Here's the drawing with two shaded views (mm, measured from the low corner). I have some questions. Coordinates: 2 decimals unless noted, no trailing zeros. Write each loop counter-clockwise with the first axis right and the second up, starting at its lowest first coordinate (ties: lowest second). Pieces come first, ordered by that corner, then holes.
Item 1: I want a section at C-C on y = 6.5. Please give me the cut outline in (x, z).
Item 2: I want a section at D-D on x = 7.75. Please give me the cut outline in (y, z), then the cut area to 3 significant figures.
Item 3: I want a section at A-A on z = 2.2. Please give me the cut outline in (x, y), then the cut area to 3 significant figures.
Item 4: For P1, Ø1.2, axis at x = 9, z = 2.5, coming from the -Y side; P2, Ø0.6, axis at y = 11.5, z = 2.5, coming from the -X side; P3, Ø0.6, axis at x = 4.5, z = 2, coming from the -Y side, each with a flat end and sliding along its axis, tell me the tip position at first contact or that it passes through.
Item 5: If I drill on probe 1 along Y at (x, z) = (3.5, 1.75); probe 2 along Z at (x, y) = (5.5, 4.5); probe 3 along X at (y, z) = (3.75, 2), over which ranges is the centre line in solid material (lowest first)?
Item 6: I want a section at B-B on x = 16. Please give me the cut outline in (y, z), then the cut area to 3 significant figures.
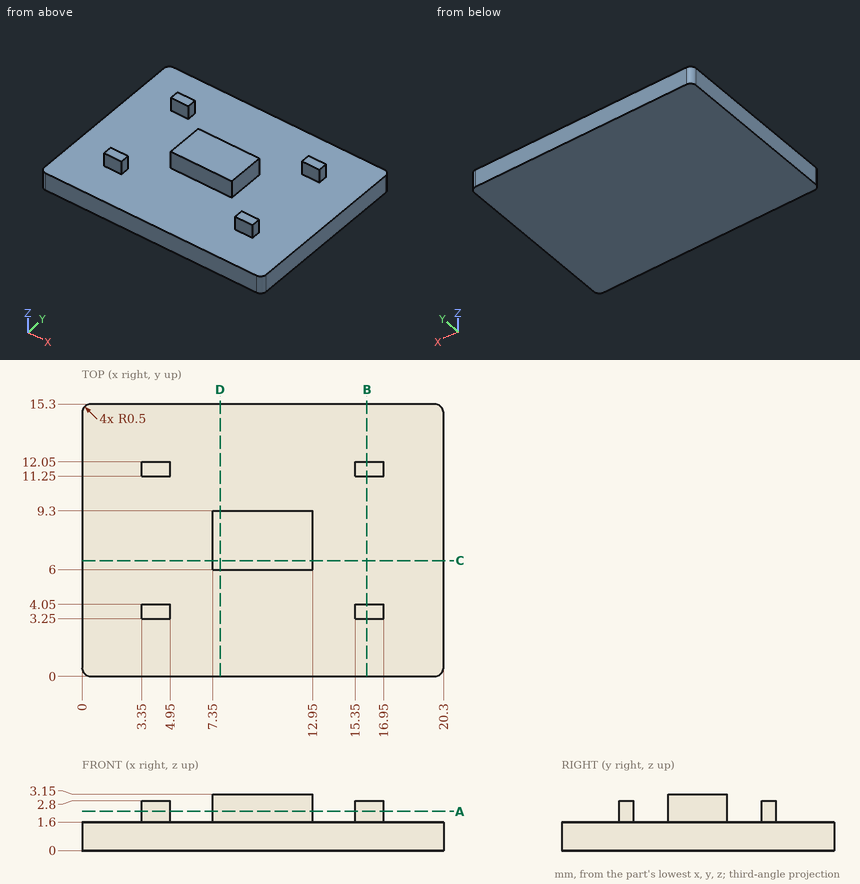
Response values:
1. outline: (0, 0) - (20.3, 0) - (20.3, 1.6) - (12.95, 1.6) - (12.95, 3.15) - (7.35, 3.15) - (7.35, 1.6) - (0, 1.6) - close
2. outline: (0, 0) - (15.3, 0) - (15.3, 1.6) - (9.3, 1.6) - (9.3, 3.15) - (6, 3.15) - (6, 1.6) - (0, 1.6) - close
2. area: 29.6 mm2
3. outline: (3.35, 3.25) - (4.95, 3.25) - (4.95, 4.05) - (3.35, 4.05) - close; (3.35, 11.25) - (4.95, 11.25) - (4.95, 12.05) - (3.35, 12.05) - close; (7.35, 6) - (12.95, 6) - (12.95, 9.3) - (7.35, 9.3) - close; (15.35, 3.25) - (16.95, 3.25) - (16.95, 4.05) - (15.35, 4.05) - close; (15.35, 11.25) - (16.95, 11.25) - (16.95, 12.05) - (15.35, 12.05) - close
3. area: 23.6 mm2
4. P1: stops at y = 6
4. P2: stops at x = 3.35
4. P3: stops at y = 3.25
5. probe 1: y = 3.25 to 4.05, 11.25 to 12.05
5. probe 2: z = 0 to 1.6
5. probe 3: x = 3.35 to 4.95, 15.35 to 16.95
6. outline: (0, 0) - (15.3, 0) - (15.3, 1.6) - (12.05, 1.6) - (12.05, 2.8) - (11.25, 2.8) - (11.25, 1.6) - (4.05, 1.6) - (4.05, 2.8) - (3.25, 2.8) - (3.25, 1.6) - (0, 1.6) - close
6. area: 26.4 mm2
